The model under review builds one solid part; all positions refer to its coordinate system, in mm. Face numbers are marked on the shaded views. A direction names the side the tool comes from. Coordinates: 2 decimals unless noted, no trailing zeros. Write each loop counter-clockwise with the first axis right and the second up, starting at its lowest first coordinate (ties: lowest second). Pieces come first, ordered by that corner, then holes. Notation, with made-up numbers: (27.5, -24) -> (79.5, -24) arc R24 cw to (79.5, 4) -> close; hole circle Ø5 at (36.25, 0.5). An arc over 180 degrees is marked (long way). Put each result on its own line as item: value. Start each with the question number.
from build123d import *

# Parameters (mm, degrees)
SKETCH1_R           = 13.5
SKETCH1_R_2         = 1.7
SKETCH1_R_3         = 5.5
BOSS_EXTRUDE1_DEPTH = 2.5
SKETCH2_R           = 13.5
SKETCH2_R_2         = 12.65
BOSS_EXTRUDE2_DEPTH = 3
SKETCH3_W           = 25
SKETCH3_H           = 25
SKETCH3_R           = 3
BOSS_EXTRUDE3_DEPTH = 4.5
CHAMFER2_SIZE       = 0.3
SKETCH4_R           = 4
BOSS_EXTRUDE4_DEPTH = 1.5
CUT_EXTRUDE1_DEPTH  = 20.868316486
CHAMFER3_SIZE       = 0.3
BOSS_EXTRUDE5_DEPTH = 4.5
CHAMFER4_SIZE       = 0.3
FILLET1_R           = 0.3
SKETCH8_R           = 1.2
CUT_EXTRUDE2_DEPTH  = 3
CHAMFER5_SIZE       = 2


with BuildPart() as part:
    # Sketch1 → Boss-Extrude1 (new body)
    with BuildSketch(Plane(origin=(0, 0, 0), x_dir=(1, 0, 0), z_dir=(0, 1, 0))):
        with Locations(Location((0, 0, 0), (0, 0, 270))):
            Circle(SKETCH1_R)
        with Locations(Location((6.646803743, 6.646803743, 0), (0, 0, 270))):
            Circle(SKETCH1_R_2, mode=Mode.SUBTRACT)
        with Locations(Location((-6.646803743, -6.646803743, 0), (0, 0, 270))):
            Circle(SKETCH1_R_2, mode=Mode.SUBTRACT)
        with Locations(Location((5.533110563, -5.533110563, 0), (0, 0, 270))):
            Circle(SKETCH1_R_2, mode=Mode.SUBTRACT)
        with Locations(Location((-5.533110563, 5.533110563, 0), (0, 0, 270))):
            Circle(SKETCH1_R_2, mode=Mode.SUBTRACT)
        with Locations(Location((0, 0, 0), (0, 0, 270))):
            Circle(SKETCH1_R_3, mode=Mode.SUBTRACT)
    extrude(amount=BOSS_EXTRUDE1_DEPTH)

    # Sketch2 → Boss-Extrude2 (add)
    with BuildSketch(Plane(origin=(0, 2.5, 0), x_dir=(1, 0, 0), z_dir=(0, 1, 0))):
        with Locations(Location((0, 0, 0), (0, 0, 270))):
            Circle(SKETCH2_R)
        with Locations(Location((0, 0, 0), (0, 0, 270))):
            Circle(SKETCH2_R_2, mode=Mode.SUBTRACT)
    extrude(amount=BOSS_EXTRUDE2_DEPTH)

    # Sketch3 → Boss-Extrude3 (add)
    with BuildSketch(Plane.XZ):
        Rectangle(SKETCH3_W, SKETCH3_H)
        with Locations(Location((-6.646803743, 6.646803743, 0), (0, 0, 270))):
            Circle(SKETCH3_R, mode=Mode.SUBTRACT)
        with Locations(Location((5.533110563, 5.533110563, 0), (0, 0, 193.381478788))):
            Circle(SKETCH3_R, mode=Mode.SUBTRACT)
        with Locations(Location((6.646803743, -6.646803743, 0), (0, 0, 270))):
            Circle(SKETCH3_R, mode=Mode.SUBTRACT)
        with Locations(Location((-5.533110563, -5.533110563, 0), (0, 0, 76.618521212))):
            Circle(SKETCH3_R, mode=Mode.SUBTRACT)
    extrude(amount=BOSS_EXTRUDE3_DEPTH)

    # Chamfer2
    chamfer2_edges = [part.edges().sort_by_distance(p)[0] for p in [
        (0, 2.5, -12.65),
    ]]
    chamfer(chamfer2_edges, length=CHAMFER2_SIZE)

    # Sketch4 → Boss-Extrude4 (add)
    # profile 1 of 3: a face of its own
    with BuildSketch(Plane(origin=(0, 0, 0), x_dir=(1, 0, 0), z_dir=(0, 1, 0))):
        with BuildLine():
            ThreePointArc((-4.838810256, 2.614558339), (-3.889087297, -3.889087297), (2.614558339, -4.838810256))
            ThreePointArc((2.614558339, -4.838810256), (3.411790219, -3.411790219), (4.838810256, -2.614558339))
            ThreePointArc((4.838810256, -2.614558339), (3.889087297, 3.889087297), (-2.614558339, 4.838810256))
            ThreePointArc((-2.614558339, 4.838810256), (-3.411790219, 3.411790219), (-4.838810256, 2.614558339))
        make_face()
        with Locations(Location((0, 0, 0), (0, 0, 270))):
            Circle(SKETCH4_R, mode=Mode.SUBTRACT)
    # profile 2 of 3: a face of its own
    with BuildSketch(Plane(origin=(0, 0, 0), x_dir=(1, 0, 0), z_dir=(0, 1, 0))):
        with BuildLine():
            ThreePointArc((-4.838810256, 2.614558339), (-3.411790219, 3.411790219), (-2.614558339, 4.838810256))
            ThreePointArc((-2.614558339, 4.838810256), (-3.889087297, 3.889087297), (-4.838810256, 2.614558339))
        make_face()
    # profile 3 of 3: a face of its own
    with BuildSketch(Plane(origin=(0, 0, 0), x_dir=(1, 0, 0), z_dir=(0, 1, 0))):
        with BuildLine():
            ThreePointArc((2.614558339, -4.838810256), (3.889087297, -3.889087297), (4.838810256, -2.614558339))
            ThreePointArc((4.838810256, -2.614558339), (3.411790219, -3.411790219), (2.614558339, -4.838810256))
        make_face()
    extrude(amount=BOSS_EXTRUDE4_DEPTH)

    # Sketch6 → Cut-Extrude1 (cut, through all)
    with BuildSketch(Plane.XZ):
        with BuildLine():
            Line((5.099019514, -12.5), (-5.099019514, -12.5))
            ThreePointArc((-5.099019514, -12.5), (0, -13.5), (5.099019514, -12.5))
        make_face()
        with BuildLine():
            Line((12.5, 5.099019514), (12.5, -5.099019514))
            ThreePointArc((12.5, -5.099019514), (13.5, 0), (12.5, 5.099019514))
        make_face()
        with BuildLine():
            Line((-5.099019514, 12.5), (5.099019514, 12.5))
            ThreePointArc((5.099019514, 12.5), (0, 13.5), (-5.099019514, 12.5))
        make_face()
        with BuildLine():
            Line((-12.5, -5.099019514), (-12.5, 5.099019514))
            ThreePointArc((-12.5, 5.099019514), (-13.5, 0), (-12.5, -5.099019514))
        make_face()
    extrude(amount=-CUT_EXTRUDE1_DEPTH, mode=Mode.SUBTRACT)

    # Chamfer3
    chamfer3_edges = [part.edges().sort_by_distance(p)[0] for p in [
        (8.944900782, 5.5, -8.944900782),
        (-8.944900782, 5.5, -8.944900782),
        (-8.944900782, 5.5, 8.944900782),
        (8.944900782, 5.5, 8.944900782),
    ]]
    chamfer(chamfer3_edges, length=CHAMFER3_SIZE)

    # Sketch7 → Boss-Extrude5 (add)
    with BuildSketch(Plane.XZ.offset(4.5)):
        Polygon((-12.5, 12.5), (-10, 12.5), (-10, 15.5), align=None)
        Polygon((-10, 12.5), (-7.5, 12.5), (-7.5, 15.5), align=None)
        Polygon((-7.5, 12.5), (-5, 12.5), (-5, 15.5), align=None)
        Polygon((-5, 12.5), (-2.5, 12.5), (-2.5, 15.5), align=None)
        Polygon((-2.5, 12.5), (0, 12.5), (0, 15.5), align=None)
        Polygon((0, 12.5), (2.5, 12.5), (2.5, 15.5), align=None)
        Polygon((2.5, 12.5), (5, 12.5), (5, 15.5), align=None)
        Polygon((5, 12.5), (7.5, 12.5), (7.5, 15.5), align=None)
        Polygon((7.5, 12.5), (10, 12.5), (10, 15.5), align=None)
        Polygon((10, 12.5), (12.5, 12.5), (12.5, 15.5), align=None)
    extrude(amount=-BOSS_EXTRUDE5_DEPTH)

    # Chamfer4
    chamfer4_edges = [part.edges().sort_by_distance(p)[0] for p in [
        (-11.25, -4.5, 14),
        (-10, -4.5, 14),
        (-7.5, -4.5, 14),
        (-8.75, -4.5, 14),
        (-5, -4.5, 14),
        (-6.25, -4.5, 14),
        (-2.5, -4.5, 14),
        (-3.75, -4.5, 14),
        (0, -4.5, 14),
        (-1.25, -4.5, 14),
        (2.5, -4.5, 14),
        (1.25, -4.5, 14),
        (5, -4.5, 14),
        (3.75, -4.5, 14),
        (7.5, -4.5, 14),
        (6.25, -4.5, 14),
        (10, -4.5, 14),
        (8.75, -4.5, 14),
        (11.25, -4.5, 14),
        (0, -4.5, -12.5),
    ]]
    chamfer(chamfer4_edges, length=CHAMFER4_SIZE)

    # Fillet1
    fillet1_edges = [part.edges().sort_by_distance(p)[0] for p in [
        (10, -2.1, 15.5),
        (7.5, -2.1, 15.5),
        (5, -2.1, 15.5),
        (2.5, -2.1, 15.5),
        (0, -2.1, 15.5),
        (-2.5, -2.1, 15.5),
        (-5, -2.1, 15.5),
        (-7.5, -2.1, 15.5),
        (-10, -2.1, 15.5),
        (12.5, -2.1, 15.5),
    ]]
    fillet(fillet1_edges, radius=FILLET1_R)

    # Sketch8 → Cut-Extrude2 (cut)
    with BuildSketch(Plane.XZ.offset(4.5)):
        with Locations(Location((0, 6, 0), (0, 0, 270))):
            Circle(SKETCH8_R)
        with Locations(Location((0, -6, 0), (0, 0, 270))):
            Circle(SKETCH8_R)
    extrude(amount=-CUT_EXTRUDE2_DEPTH, mode=Mode.SUBTRACT)

    # Chamfer5
    # the kernel refuses this chamfer: 2 mm, written as the material it adds along each edge
    with BuildSketch(Plane(origin=(-5.533110563, 0, -5.533110563), x_dir=(0.2314334356248564, 0, 0.9728507413138335), z_dir=(0.9728507413138335, 0, -0.2314334356248564))) as chamfer5_piece_1_section:
        Polygon((3, CHAMFER5_SIZE), (3 - CHAMFER5_SIZE, 0), (3, 0), align=None)
    chamfer5_piece_1 = revolve(axis=Axis((-5.533110563, 0, -5.533110563), (0, -1, 0)), mode=Mode.PRIVATE)
    chamfer5_piece_1 = chamfer5_piece_1 - Plane(origin=(-5.533110563, -1.35638922, -5.533110563), x_dir=(0, 0, 1), z_dir=(0, -1, 0)) * Cylinder(1.7, 13, mode=Mode.PRIVATE)
    add(chamfer5_piece_1)
    with BuildSketch(Plane(origin=(5.533110563, 0, 5.533110563), x_dir=(-0.9728507413138336, 0, -0.23143343562485635), z_dir=(-0.23143343562485635, 0, 0.9728507413138336))) as chamfer5_piece_2_section:
        Polygon((3, CHAMFER5_SIZE), (3 - CHAMFER5_SIZE, 0), (3, 0), align=None)
    chamfer5_piece_2 = revolve(axis=Axis((5.533110563, 0, 5.533110563), (0, -1, 0)), mode=Mode.PRIVATE)
    chamfer5_piece_2 = chamfer5_piece_2 - Plane(origin=(5.533110563, -1.35638922, 5.533110563), x_dir=(0, 0, 1), z_dir=(0, -1, 0)) * Cylinder(1.7, 12, mode=Mode.PRIVATE)
    add(chamfer5_piece_2)
    with BuildSketch(Plane(origin=(6.646803743, 0, -6.646803743), x_dir=(0, 0, -1), z_dir=(-1, 0, 0))) as chamfer5_piece_3_section:
        Polygon((3, CHAMFER5_SIZE), (3 - CHAMFER5_SIZE, 0), (3, 0), align=None)
    chamfer5_piece_3 = revolve(axis=Axis((6.646803743, 0, -6.646803743), (0, -1, 0)), mode=Mode.PRIVATE)
    chamfer5_piece_3 = chamfer5_piece_3 - Plane(origin=(6.646803743, -1.35638922, -6.646803743), x_dir=(0, 0, 1), z_dir=(0, -1, 0)) * Cylinder(1.7, 13, mode=Mode.PRIVATE)
    add(chamfer5_piece_3)
    with BuildSketch(Plane(origin=(-6.646803743, 0, 6.646803743), x_dir=(0, 0, -1), z_dir=(-1, 0, 0))) as chamfer5_piece_4_section:
        Polygon((3, CHAMFER5_SIZE), (3 - CHAMFER5_SIZE, 0), (3, 0), align=None)
    chamfer5_piece_4 = revolve(axis=Axis((-6.646803743, 0, 6.646803743), (0, -1, 0)), mode=Mode.PRIVATE)
    chamfer5_piece_4 = chamfer5_piece_4 - Plane(origin=(-6.646803743, -1.35638922, 6.646803743), x_dir=(0, 0, 1), z_dir=(0, -1, 0)) * Cylinder(1.7, 13, mode=Mode.PRIVATE)
    add(chamfer5_piece_4)


solid = part.part
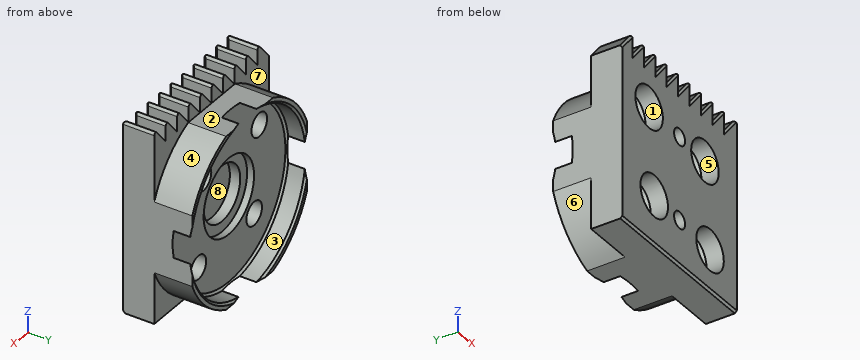
1. Wall thickness on line 1 (X direction, y = 0.75, z = -3.5); line 2 (Z direction, x = 5.5, y = -2.75); line 3 (Z direction, x = 7.25, y = -1): over which ranges is each line inside the solid? List them lowest first. Write a range as from..to.
2. Consider section A-A on y = 3.5. State the section outline as (x, z) points.
3. The part is to be moulded in two halves that separate along Z. For the marked faces 5, 6, 7 and 8, say which applies: released by +Z, released by -Z, zero draft, split by the parting line, or undercut.
4. Insertion check: P1, Ø0.7, axis at x = 4, z = 13.5, coming from the +Y side; P2, Ø4.5, axis at x = -6.65, z = 6.65, coming from the -Y side; P3, Ø5.5, axis at x = -5.53, z = -5.53, coming from the -Y side. Each pin has a flat end and moves straight along its axis. Give the tip position at first contact, or say it passes through.
5. Tool access review of the marked faces 1, 2, 3 and 4: name each direction out of +Z, -Z, +X, -X, +Y, -Y from which nothing blocks a thin tool from reaching the whole face with its end or side.
6. Consider section B-B on z = 0. State the section outline as (x, y) points, then the cut area to 3 significant figures.
7. Consider section C-C on z = -6. State how many separate pieces and enclosed holes the cut face has, then the cut area to 3 significant figures.
Output values:
1. line 1: x = -12.5..-1.94, 1.94..12.5
1. line 2: z = -12.5..-9.42, -3.87..2.53, 8.53..13.1
1. line 3: z = -12.5..-8.55, -4.74..4.51, 6.56..14.97
2. outline: (-12.5, -5.1) arc R13.5 ccw to (-5.1, -12.5) -> (-1.94, -12.5) arc R12.65 cw to (-12.5, -1.94) -> close; (-12.5, 1.94) arc R12.65 cw to (-1.94, 12.5) -> (-5.1, 12.5) arc R13.5 ccw to (-12.5, 5.1) -> close; (1.94, -12.5) -> (5.1, -12.5) arc R13.5 ccw to (12.5, -5.1) -> (12.5, -1.94) arc R12.65 cw to start; (1.94, 12.5) arc R12.65 cw to (12.5, 1.94) -> (12.5, 5.1) arc R13.5 ccw to (5.1, 12.5) -> close
3. face 5: undercut
3. face 6: released by -Z
3. face 7: zero draft
3. face 8: undercut
4. P1: stops at y = 0
4. P2: stops at y = -1.25
4. P3: stops at y = -1.75
5. face 1: -Y
5. face 2: +Z, +X, -X, +Y
5. face 3: +Y
5. face 4: +Z, +X, +Y
6. outline: (-12.5, -4.5) -> (12.5, -4.5) -> (12.5, 2.65) -> (12.35, 2.5) -> (5.5, 2.5) -> (5.5, 1.5) -> (4, 1.5) -> (4, 0) -> (-4, 0) -> (-4, 1.5) -> (-5.5, 1.5) -> (-5.5, 2.5) -> (-12.35, 2.5) -> (-12.5, 2.65) -> close
6. area: 152 mm^2
7. separate pieces: 3
7. enclosed holes: 0
7. area: 110 mm^2
